from build123d import *

# Parameters (mm, degrees)
BOSS_EXTRUDE1_DEPTH = 35.814
CUT_EXTRUDE1_DEPTH  = 30.734
SKETCH5_R           = 3.937
CUT_EXTRUDE2_DEPTH  = 12.7
SKETCH7_W           = 137.16
SKETCH7_H           = 17.907
CUT_EXTRUDE3_DEPTH  = 5.08
SKETCH8_W           = 90.016933803
SKETCH8_H           = 17.907
CUT_EXTRUDE4_DEPTH  = 5.08


with BuildPart() as part:
    # Sketch1 → Boss-Extrude1 (new body)
    with BuildSketch(Plane(origin=(0, 0, 0), x_dir=(1, 0, 0), z_dir=(0, 1, 0))):
        with BuildLine():
            Line((94.928870908, -1.703626264), (55.529419709, 56.18731626))
            ThreePointArc((55.529419709, 56.18731626), (41.967930942, 66.402029849), (24.990687805, 66.235997574))
            Line((24.990687805, 66.235997574), (-71.166136997, 14.689688471))
            Line((-71.166136997, 14.689688471), (-24.920143323, -68.405045948))
            Line((-24.920143323, -68.405045948), (94.928870908, -1.703626264))
        make_face()
    extrude(amount=BOSS_EXTRUDE1_DEPTH)

    # Sketch1_6 → Cut-Extrude1 (cut)
    with BuildSketch(Plane(origin=(0, 0, 0), x_dir=(1, 0, 0), z_dir=(0, 1, 0))):
        with BuildLine():
            Line((26.052021788, 63.812159478), (-67.558235137, 13.630976306))
            Line((-67.558235137, 13.630976306), (-23.898074198, -64.817537603))
            Line((-23.898074198, -64.817537603), (91.124715274, -0.802131195))
            Line((91.124715274, -0.802131195), (53.348830885, 54.703249855))
            ThreePointArc((53.348830885, 54.703249855), (41.23793969, 63.8651945), (26.052021788, 63.812159478))
        make_face()
    extrude(amount=CUT_EXTRUDE1_DEPTH, mode=Mode.SUBTRACT)

    # Sketch5 → Cut-Extrude2 (cut)
    with BuildSketch(Plane(origin=(0, 35.814, 0), x_dir=(1, 0, 0), z_dir=(0, 1, 0))):
        with Locations((-11.924156141, 0.45361366)):
            Circle(SKETCH5_R)
    extrude(amount=-CUT_EXTRUDE2_DEPTH, mode=Mode.SUBTRACT)

    # Sketch7 → Cut-Extrude3 (cut)
    with BuildSketch(Plane(origin=(23.173771068, 0, 41.638598275), x_dir=(0.873789838, 0, -0.486303731), z_dir=(0.486303731, 0, 0.873789838))):
        with Locations((13.53940296, 8.9535)):
            Rectangle(SKETCH7_W, SKETCH7_H)
    extrude(amount=-CUT_EXTRUDE3_DEPTH, mode=Mode.SUBTRACT)

    # Sketch8 → Cut-Extrude4 (cut)
    with BuildSketch(Plane(origin=(-48.093914392, 0, 26.766447673), x_dir=(0.486303731, 0, 0.873789838), z_dir=(-0.873789838, 0, 0.486303731))):
        with Locations((-2.435591524, 8.9535)):
            Rectangle(SKETCH8_W, SKETCH8_H)
    extrude(amount=-CUT_EXTRUDE4_DEPTH, mode=Mode.SUBTRACT)


solid = part.part
Input: part model. Units: mm. Frame: model coordinates. A direction names the side the tool comes from. Coordinates: 2 decimals unless noted, no trailing zeros. Loops run counter-clockwise (first coordinate to the right, second up) from the corner with the lowest first, then second, coordinate; pieces in that order, holes last.
Q1. Cut plane A-A (y = 5). Output: boundary loops of the cut face in (x, z).
Q2. Material intervals for line 1 (Y direction, x = -53, z = -16); line 2 (X direction, y = 28.5, z = -37); line 3 (X direction, y = 6, z = -54), sorted ascending.
Q3. Set-up query: faces 4 (the face through (32.808, 24.231, 33.258)), 5 (the face through (75.505, 17.656, -26.837)). Return all of +Z, -Z, +X, -X, +Y, -Y with unobstructed straight access to the full face (end or side cutting, diameter ignored); none if empty.
Q4. Draft query along Z for faces 1 (the face through (11, 35.814, -1)), 2 (the face through (-22.415, 17.656, -40.824)), 3 (the face through (11, 30.734, -1)). Return one class per face: +Z half, -Z half, draft (parallel to the pull), parting line (faces both ways), or undercut.
Q5. Contact query for flat-ended pins moving along their axis: pin 1 (12 mm diameter, centred on x = 60.5, y = 8, fed in from +Z); pin 2 (1.5 mm diameter, centred on y = 25.5, z = -12.5, fed in from -X); pin 3 (3 mm diameter, centred on x = -28, z = -31, fed in from -Y). Output: stop coordinate, or through.
Q6. Cut plane B-B (y = 27.5). Output: boundary loops of the cut face in (x, z).
Q7. Cut plane C-C (z = 38). Output: boundary loops of the cut face in (x, y), then the cut area to 3 significant figures.
Working result:
1. outline: (-66.69, -17.09) - (24.99, -66.24) arc R26.38 ccw to (55.53, -56.19) - (92.06, -2.51) - (89.75, -1.23) - (53.35, -54.7) arc R23.74 cw to (26.05, -63.81) - (-65.41, -14.79) - close
2. line 1: y = 30.73 to 35.81
2. line 2: x = -29.55 to -23.96, 65.4 to 68.59
2. line 3: x = 2.17 to 7.75, 53.83 to 57.02
3. face 4: -Y
3. face 5: -Z, +X, +Y, -Y
4. face 1: draft
4. face 2: -Z half
4. face 3: undercut
5. pin 1: stops at z = -35.38
5. pin 2: stops at x = -70.36
5. pin 3: stops at y = 30.73
6. outline: (-71.17, -14.69) - (24.99, -66.24) arc R26.38 ccw to (55.53, -56.19) - (94.93, 1.7) - (-24.92, 68.41) - close; hole (-67.56, -13.63) - (26.05, -63.81) arc R23.74 ccw to (53.35, -54.7) - (91.12, 0.8) - (-23.9, 64.82) - close
7. outline: (-41.84, 17.91) - (-38.82, 17.91) - (-38.82, 30.73) - (24.29, 30.73) - (24.29, 17.91) - (29.71, 17.91) - (29.71, 35.81) - (-41.84, 35.81) - close
7. area: 472 mm2
